Work out the finished part from the listing and answer in its coordinate system (mm). A direction names the side the tool comes from. Coordinates: 2 decimals unless noted, no trailing zeros. Loops run counter-clockwise (first coordinate to the right, second up) from the corner with the lowest first, then second, coordinate; pieces in that order, holes last. Notation, with made-up numbers: (-4.75, -20.75) - (33.25, -20.75) arc R25 ccw to (33.25, 13.25) - close; hole circle Ø6 at (63.25, 69). An arc over 180 degrees is marked (long way). Write each question's results on one line, items separated by ' | '. Start each with the question number.
1. A cutting plane is placed at B-B on y = 15. Determine the outline of the cut face in (x, z), then the cut area to 3 significant figures.
2. Which of the six approach directions +Z, -Z, +X, -X, +Y, -Y give full straight-line access (tool end or side, diameter ignored) to faces 5 (the flat face through (9, -76, 15.5)), 6 (the flat face through (6, 35, 27)), 7 (the cylindrical face through (5.92, -37.57, 8.11)), 8 (the flat face through (5, 71, -18)), 9 (the cylindrical face through (6, -79, 11))?
3. A cutting plane is placed at A-A on y = -45. Determine the outline of the cut face in (x, z), then the cut area to 3 significant figures.
4. Determine the mould class of faces 1 (the flat face through (2, 74, 47)), 2 (the flat face through (6, -93, 0)), 3 (the flat face through (6, -1, -27)), 4 (the flat face through (5.5, 76, 18)) for opening direction Z: released by +Z, released by -Z, zero draft, split by the parting line, or undercut.
5. A cutting plane is placed at C-C on z = 0. State how many separate pieces and enclosed holes the cut face has, then the cut area to 3 significant figures.
6. Each of these flat-tipped pins is pushed along its axis until it touches: P1, Ø6, axis at x = 4.5, z = 34.5, coming from the +Y side; P2, Ø13, axis at y = 45, z = 0, coming from the -X side; P3, Ø1.2, axis at x = 1, z = 40, coming from the -Y side; P4, Ø4, axis at x = 9, y = -20.5, coming from the +Z side. Where does it stop, or does it pass through?
7. Find the intervals of material crossed by line 1 along Z through (x, y) = (2.2, 74); line 2 along Z through (x, y) = (5.75, -76.5); line 3 along Y through (x, z) = (2.75, -4), in increasing order. Write a range as [from, to].
from build123d import *

# Parameters (mm, degrees)
SKETCH2_W                    = 54
SKETCH2_H                    = 162
SKETCH2_R                    = 10.5
SKETCH2_R_2                  = 11
BOSS_EXTRUDE1_DEPTH          = 12
SKETCH3_W                    = 18
SKETCH3_H                    = 12
BOSS_EXTRUDE2_DEPTH          = 12
CUT_EXTRUDE1_REACH           = 99.581
SKETCH4_R                    = 2.25
LPATTERN1_COUNT              = 2
LPATTERN1_PITCH              = 90
CUT_EXTRUDE14_START          = 4
CUT_EXTRUDE14_DEPTH          = 8
CUT_EXTRUDE15_DEPTH          = 6.5
MIRROR2_START                = 4
MIRROR2_COPY_1_DEPTH         = 8
MIRROR2_COPY_2_DEPTH         = 6.5
CUT_EXTRUDE9_REACH           = 99.581
SKETCH13_R                   = 2.5
SKETCH15_W                   = 20
SKETCH15_H                   = 15
BOSS_EXTRUDE3_DEPTH          = 12
F_2_0_2_DIAMETER_HOLE1_D     = 2
SKETCH19_W                   = 10
SKETCH19_H                   = 70
BOSS_EXTRUDE4_DEPTH          = 12
F_2_0_2_DIAMETER_HOLE2_D     = 2
CUT_EXTRUDE12_REACH          = 110.89
CUT_EXTRUDE12_START          = -4
SKETCH22_W                   = 20
SKETCH22_H                   = 15
FILLET1_R                    = 2
CUT_EXTRUDE13_REACH          = 106.89
F_5_0_5_DIAMETER_HOLE2_D     = 5
F_5_0_5_DIAMETER_HOLE1_D     = 5
F_5_0_5_DIAMETER_HOLE1_DEPTH = 12
F_5_0_5_DIAMETER_HOLE1_TIP   = 1.502151548
SKETCH32_W                   = 4
SKETCH32_H                   = 8
CUT_EXTRUDE16_DEPTH          = 3
FILLET2_R                    = 2


# Read off the part's stored shape, not the designer's step: Cut-Extrude14
with BuildPart() as part:
    # Sketch2 → Boss-Extrude1 (new body)
    with BuildSketch(Plane(origin=(0, 0, 0), x_dir=(0, 0, -1), z_dir=(1, 0, 0))):
        Rectangle(SKETCH2_W, SKETCH2_H)
        Circle(SKETCH2_R, mode=Mode.SUBTRACT)
        with Locations((0, 45)):
            Circle(SKETCH2_R_2, mode=Mode.SUBTRACT)
        with Locations((0, -45)):
            Circle(SKETCH2_R_2, mode=Mode.SUBTRACT)
    extrude(amount=BOSS_EXTRUDE1_DEPTH)

    # Sketch3 → Boss-Extrude2 (add)
    with BuildSketch(Plane(origin=(12, 0, 0), x_dir=(0, 0, -1), z_dir=(1, 0, 0))):
        with Locations((0, -87)):
            Rectangle(SKETCH3_W, SKETCH3_H)
    boss_extrude2 = extrude(amount=-BOSS_EXTRUDE2_DEPTH)

    # Mirror1: Boss-Extrude2 across plane
    add(boss_extrude2.mirror(Plane.ZX))

    # Sketch4 → Cut-Extrude1 (cut, up to next)
    with BuildSketch(Plane(origin=(12, 0, 0), x_dir=(0, 0, -1), z_dir=(1, 0, 0)), mode=Mode.PRIVATE) as cut_extrude1_sk1:
        with Locations((-16, -45)):
            Circle(SKETCH4_R)
    cut_extrude1_tool1 = extrude(cut_extrude1_sk1.sketch, amount=-CUT_EXTRUDE1_REACH, mode=Mode.PRIVATE) & part.part
    # Sketch4 → Cut-Extrude1 (cut, up to next)
    with BuildSketch(Plane(origin=(12, 0, 0), x_dir=(0, 0, -1), z_dir=(1, 0, 0)), mode=Mode.PRIVATE) as cut_extrude1_sk2:
        with Locations((16, -45)):
            Circle(SKETCH4_R)
    cut_extrude1_tool2 = extrude(cut_extrude1_sk2.sketch, amount=-CUT_EXTRUDE1_REACH, mode=Mode.PRIVATE) & part.part
    cut_extrude1_1 = cut_extrude1_tool1.solids().sort_by_distance((12, -45, 16))[0]
    add(cut_extrude1_1, mode=Mode.SUBTRACT)
    cut_extrude1_2 = cut_extrude1_tool2.solids().sort_by_distance((12, -45, -16))[0]
    add(cut_extrude1_2, mode=Mode.SUBTRACT)
    cut_extrude1 = cut_extrude1_1 + cut_extrude1_2  # Cut-Extrude1 as one shape, for the pattern or mirror that repeats it

    # LPattern1: Cut-Extrude1 ×2
    with Locations(*[(0, i * LPATTERN1_PITCH, 0) for i in range(1, LPATTERN1_COUNT)]):
        add(cut_extrude1, mode=Mode.SUBTRACT)

    # Cut-Extrude14 outline → Cut-Extrude14 (cut)
    with BuildSketch(Plane.YZ.offset(CUT_EXTRUDE14_START)):
        with BuildLine():
            Line((71, -22), (71, -14))
            ThreePointArc((71, -14), (69, -12), (67, -14))
            Line((67, -14), (67, -22))
            ThreePointArc((67, -22), (69, -24), (71, -22))
        make_face()
    cut_extrude14 = extrude(amount=CUT_EXTRUDE14_DEPTH, mode=Mode.SUBTRACT)

    # Sketch27 → Cut-Extrude15 (cut)
    with BuildSketch(Plane(origin=(12, 165.584173165, 19.767626803), x_dir=(0, 0, -1), z_dir=(1, 0, 0))):
        with BuildLine():
            Line((40.267626803, -47.95431377), (40.267626803, -101.584173165))
            ThreePointArc((40.267626803, -101.584173165), (37.767626803, -104.084173165), (35.267626803, -101.584173165))
            Line((35.267626803, -101.584173165), (35.267626803, -47.95431377))
            ThreePointArc((35.267626803, -47.95431377), (37.767626803, -45.45431377), (40.267626803, -47.95431377))
        make_face()
    cut_extrude15 = extrude(amount=-CUT_EXTRUDE15_DEPTH, mode=Mode.SUBTRACT)

    # Mirror3: Cut-Extrude14, Cut-Extrude15 across plane
    add(cut_extrude14.mirror(Plane.XY), mode=Mode.SUBTRACT)
    add(cut_extrude15.mirror(Plane.XY), mode=Mode.SUBTRACT)

    # Mirror2: Cut-Extrude14, Cut-Extrude15 across plane
    add(cut_extrude14.mirror(Plane.ZX), mode=Mode.SUBTRACT)
    add(cut_extrude15.mirror(Plane.ZX), mode=Mode.SUBTRACT)

    # Mirror2 copy 1 sketch → Mirror2 copy 1 (cut)
    with BuildSketch(Plane(origin=(0, 0, 0), x_dir=(0, -1, 0), z_dir=(1, 0, 0)).offset(MIRROR2_START)):
        with BuildLine():
            Line((71, -22), (71, -14))
            ThreePointArc((71, -14), (69, -12), (67, -14))
            Line((67, -14), (67, -22))
            ThreePointArc((67, -22), (69, -24), (71, -22))
        make_face()
    extrude(amount=MIRROR2_COPY_1_DEPTH, mode=Mode.SUBTRACT)

    # Mirror2 copy 2 sketch → Mirror2 copy 2 (cut)
    with BuildSketch(Plane(origin=(12, -165.584173165, -19.767626803), x_dir=(0, 0, 1), z_dir=(1, 0, 0))):
        with BuildLine():
            Line((40.267626803, -47.95431377), (40.267626803, -101.584173165))
            ThreePointArc((40.267626803, -101.584173165), (37.767626803, -104.084173165), (35.267626803, -101.584173165))
            Line((35.267626803, -101.584173165), (35.267626803, -47.95431377))
            ThreePointArc((35.267626803, -47.95431377), (37.767626803, -45.45431377), (40.267626803, -47.95431377))
        make_face()
    extrude(amount=-MIRROR2_COPY_2_DEPTH, mode=Mode.SUBTRACT)

    # Sketch13 → Cut-Extrude9 (cut, up to next)
    with BuildSketch(Plane.ZY, mode=Mode.PRIVATE) as cut_extrude9_sk1:
        with Locations((0, 15)):
            Circle(SKETCH13_R)
    cut_extrude9_tool1 = extrude(cut_extrude9_sk1.sketch, amount=-CUT_EXTRUDE9_REACH, mode=Mode.PRIVATE) & part.part
    # Sketch13 → Cut-Extrude9 (cut, up to next)
    with BuildSketch(Plane.ZY, mode=Mode.PRIVATE) as cut_extrude9_sk2:
        with Locations((0, -15)):
            Circle(SKETCH13_R)
    cut_extrude9_tool2 = extrude(cut_extrude9_sk2.sketch, amount=-CUT_EXTRUDE9_REACH, mode=Mode.PRIVATE) & part.part
    add(cut_extrude9_tool1.solids().sort_by_distance((0, 15, 0))[0], mode=Mode.SUBTRACT)
    add(cut_extrude9_tool2.solids().sort_by_distance((0, -15, 0))[0], mode=Mode.SUBTRACT)

    # Sketch15 → Boss-Extrude3 (add)
    with BuildSketch(Plane.ZY):
        with Locations((37, 73.5)):
            Rectangle(SKETCH15_W, SKETCH15_H)
    extrude(amount=-BOSS_EXTRUDE3_DEPTH)

    # Ø2.0 (2) Diameter Hole1 (through all)
    with Locations(Plane(origin=(12, 0, 0), x_dir=(0, 0, -1), z_dir=(1, 0, 0))):
        with Locations((-41.5, 74), (-32, 74)):
            Hole(F_2_0_2_DIAMETER_HOLE1_D / 2)

    # Sketch19 → Boss-Extrude4 (add)
    with BuildSketch(Plane.ZY):
        with Locations((32, -46)):
            Rectangle(SKETCH19_W, SKETCH19_H)
    extrude(amount=-BOSS_EXTRUDE4_DEPTH)

    # Ø2.0 (2) Diameter Hole2 (through all)
    with Locations(Plane(origin=(12, 0, 0), x_dir=(0, 0, -1), z_dir=(1, 0, 0))):
        with Locations((-31.5, -19), (-22, -19)):
            Hole(F_2_0_2_DIAMETER_HOLE2_D / 2)

    # Sketch22 → Cut-Extrude12 (cut, up to next)
    with BuildSketch(Plane.ZY.offset(CUT_EXTRUDE12_START), mode=Mode.PRIVATE) as cut_extrude12_sk1:
        with Locations((37, 73.5)):
            Rectangle(SKETCH22_W, SKETCH22_H)
    cut_extrude12_tool1 = extrude(cut_extrude12_sk1.sketch, amount=-CUT_EXTRUDE12_REACH, mode=Mode.PRIVATE) & part.part
    # Sketch22 → Cut-Extrude12 (cut, up to next)
    with BuildSketch(Plane.ZY.offset(CUT_EXTRUDE12_START), mode=Mode.PRIVATE) as cut_extrude12_sk2:
        Polygon((15, -11), (27, -6.632357189), (37, -11), (37, -27), (15, -27), align=None)
    cut_extrude12_tool2 = extrude(cut_extrude12_sk2.sketch, amount=-CUT_EXTRUDE12_REACH, mode=Mode.PRIVATE) & part.part
    add(cut_extrude12_tool1.solids().sort_by_distance((4, 73.5, 37))[0], mode=Mode.SUBTRACT)
    add(cut_extrude12_tool2.solids().sort_by_distance((4, -17.864378, 26.040032))[0], mode=Mode.SUBTRACT)

    # Fillet1
    fillet1_edges = [part.edges().sort_by_distance(p)[0] for p in [
        (8, -11, 15),
        (8, -27, 15),
        (2, 66, 27),
        (2, -11, 27),
        (2, 66, 47),
        (2, -11, 37),
        (8, -27, 37),
    ]]
    fillet(fillet1_edges, radius=FILLET1_R)

    # Sketch23 → Cut-Extrude13 (cut, up to next)
    with BuildSketch(Plane.ZY, mode=Mode.PRIVATE) as cut_extrude13_sk1:
        with BuildLine():
            Line((-13, 81), (-9, 81))
            ThreePointArc((-9, 81), (-11, 79), (-13, 81))
        make_face()
    cut_extrude13_tool1 = extrude(cut_extrude13_sk1.sketch, amount=-CUT_EXTRUDE13_REACH, mode=Mode.PRIVATE) & part.part
    # Sketch23 → Cut-Extrude13 (cut, up to next)
    with BuildSketch(Plane.ZY, mode=Mode.PRIVATE) as cut_extrude13_sk2:
        with BuildLine():
            Line((9, 81), (13, 81))
            ThreePointArc((13, 81), (11, 79), (9, 81))
        make_face()
    cut_extrude13_tool2 = extrude(cut_extrude13_sk2.sketch, amount=-CUT_EXTRUDE13_REACH, mode=Mode.PRIVATE) & part.part
    # Sketch23 → Cut-Extrude13 (cut, up to next)
    with BuildSketch(Plane.ZY, mode=Mode.PRIVATE) as cut_extrude13_sk3:
        with BuildLine():
            Line((-13, -81), (-9, -81))
            ThreePointArc((-9, -81), (-11, -79), (-13, -81))
        make_face()
    cut_extrude13_tool3 = extrude(cut_extrude13_sk3.sketch, amount=-CUT_EXTRUDE13_REACH, mode=Mode.PRIVATE) & part.part
    # Sketch23 → Cut-Extrude13 (cut, up to next)
    with BuildSketch(Plane.ZY, mode=Mode.PRIVATE) as cut_extrude13_sk4:
        with BuildLine():
            Line((9, -81), (13, -81))
            ThreePointArc((13, -81), (11, -79), (9, -81))
        make_face()
    cut_extrude13_tool4 = extrude(cut_extrude13_sk4.sketch, amount=-CUT_EXTRUDE13_REACH, mode=Mode.PRIVATE) & part.part
    add(cut_extrude13_tool1.solids().sort_by_distance((0, 80.151174, -11))[0], mode=Mode.SUBTRACT)
    add(cut_extrude13_tool2.solids().sort_by_distance((0, 80.151174, 11))[0], mode=Mode.SUBTRACT)
    add(cut_extrude13_tool3.solids().sort_by_distance((0, -80.151174, -11))[0], mode=Mode.SUBTRACT)
    add(cut_extrude13_tool4.solids().sort_by_distance((0, -80.151174, 11))[0], mode=Mode.SUBTRACT)

    # Ø5.0 (5) Diameter Hole2 (through all)
    with Locations(Plane(origin=(12, 0, 0), x_dir=(0, 0, -1), z_dir=(1, 0, 0))):
        with Locations((0, -26), (0, 26)):
            Hole(F_5_0_5_DIAMETER_HOLE2_D / 2)

    # Ø5.0 (5) Diameter Hole1
    with Locations(Plane.ZY):
        with Locations((0, 85), (0, -85)):
            Hole(F_5_0_5_DIAMETER_HOLE1_D / 2, depth=F_5_0_5_DIAMETER_HOLE1_DEPTH)
            with Locations((0, 0, -(F_5_0_5_DIAMETER_HOLE1_DEPTH + F_5_0_5_DIAMETER_HOLE1_TIP / 2))):  # 118° drill point
                Cone(0, F_5_0_5_DIAMETER_HOLE1_D / 2, F_5_0_5_DIAMETER_HOLE1_TIP, mode=Mode.SUBTRACT)

    # Sketch32 → Cut-Extrude16 (cut)
    with BuildSketch(Plane(origin=(12, 0, 0), x_dir=(0, 0, -1), z_dir=(1, 0, 0))):
        with Locations((-25, 77)):
            Rectangle(SKETCH32_W, SKETCH32_H)
    extrude(amount=-CUT_EXTRUDE16_DEPTH, mode=Mode.SUBTRACT)

    # Fillet2
    fillet2_edges = [part.edges().sort_by_distance(p)[0] for p in [
        (10.5, 73, 23),
    ]]
    fillet(fillet2_edges, radius=FILLET2_R)


solid = part.part
Values:
1) outline: (0, -27) - (12, -27) - (12, -2.5) - (0, -2.5) - close; (0, 2.5) - (12, 2.5) - (12, 27) - (0, 27) - close | area: 588 mm^2
2) face 5: +X, -Y | face 6: +Z, +X | face 7: +X, -X | face 8: +X | face 9: +X, -X, -Y
3) outline: (0, -27) - (12, -27) - (12, -18.25) - (0, -18.25) - close; (0, -13.75) - (12, -13.75) - (12, -11) - (0, -11) - close; (0, 11) - (12, 11) - (12, 13.75) - (0, 13.75) - close; (0, 18.25) - (12, 18.25) - (12, 37) - (0, 37) - close | area: 396 mm^2
4) face 1: released by +Z | face 2: zero draft | face 3: released by -Z | face 4: undercut
5) separate pieces: 10 | enclosed holes: 0 | area: 1,090 mm^2
6) P1: y = 81 | P2: through | P3: y = 66 | P4: z = 15
7) line 1: [-27, 31], [33, 40.5], [42.5, 47] | line 2: [-27, -20.5], [-15.5, 15.5], [20.5, 37] | line 3: [-93, -55.25], [-34.75, -9.71], [9.71, 34.75], [55.25, 93]
